from build123d import *

# Parameters (mm, degrees)
SKETCH1_W           = 116
SKETCH1_H           = 90
BOSS_EXTRUDE1_DEPTH = 5
SKETCH2_W           = 5
SKETCH2_H           = 90
BOSS_EXTRUDE2_DEPTH = 120
SKETCH3_R           = 40
CUT_EXTRUDE1_DEPTH  = 15
SKETCH4_R           = 2.5
CUT_EXTRUDE2_DEPTH  = 15
SKETCH5_W           = 5
SKETCH5_H           = 90
BOSS_EXTRUDE3_DEPTH = 120


with BuildPart() as part:
    # Sketch1 → Boss-Extrude1 (new body)
    with BuildSketch(Plane(origin=(0, 0, 0), x_dir=(1, 0, 0), z_dir=(0, 1, 0))):
        with Locations((58, 45)):
            Rectangle(SKETCH1_W, SKETCH1_H)
    extrude(amount=BOSS_EXTRUDE1_DEPTH)

    # Sketch2 → Boss-Extrude2 (add)
    with BuildSketch(Plane(origin=(0, 5, 0), x_dir=(1, 0, 0), z_dir=(0, 1, 0))):
        with Locations((113.5, 45)):
            Rectangle(SKETCH2_W, SKETCH2_H)
    extrude(amount=BOSS_EXTRUDE2_DEPTH)

    # Sketch3 → Cut-Extrude1 (cut)
    with BuildSketch(Plane.XZ):
        with Locations(Location((68, -45, 0), (0, 0, 270))):
            Circle(SKETCH3_R)
    extrude(amount=-CUT_EXTRUDE1_DEPTH, mode=Mode.SUBTRACT)

    # Sketch4 → Cut-Extrude2 (cut)
    with BuildSketch(Plane.XZ):
        with Locations(Location((32, -9, 0), (0, 0, 270))):
            Circle(SKETCH4_R)
        with Locations(Location((104, -9, 0), (0, 0, 270))):
            Circle(SKETCH4_R)
        with Locations(Location((104, -81, 0), (0, 0, 270))):
            Circle(SKETCH4_R)
        with Locations(Location((32, -81, 0), (0, 0, 270))):
            Circle(SKETCH4_R)
    extrude(amount=-CUT_EXTRUDE2_DEPTH, mode=Mode.SUBTRACT)

    # Sketch5 → Boss-Extrude3 (add)
    with BuildSketch(Plane(origin=(0, 5, 0), x_dir=(1, 0, 0), z_dir=(0, 1, 0))):
        with Locations((22.5, 45)):
            Rectangle(SKETCH5_W, SKETCH5_H)
    extrude(amount=BOSS_EXTRUDE3_DEPTH)


solid = part.part
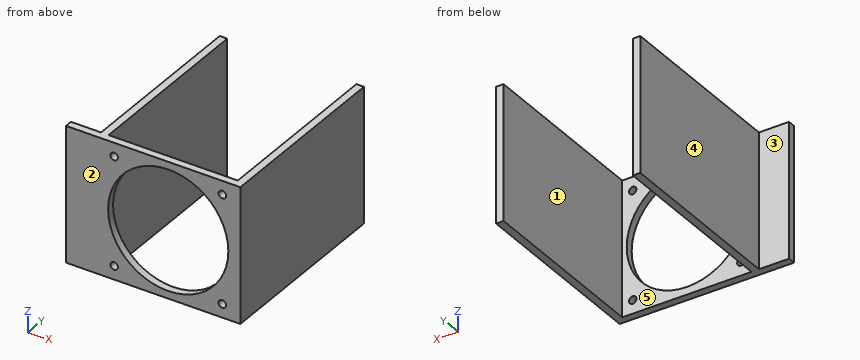
Can you work these out from the model? Positions are in its coordinate system, mm. Face numbers are marked on the shaded views. A direction names the side the tool comes from. Coordinates: 2 decimals unless noted, no trailing zeros. Loops run counter-clockwise (first coordinate to the right, second up) from the corner with the lowest first, then second, coordinate; pieces in that order, holes last. Notation, with made-up numbers: M 3.25,-35.75 L 29.25,-35.75 A20 cw 29.25,0.25 Z; hole C -7.75,82 d3. An arc over 180 degrees is marked long. Return JSON: item names as keys, results as strings. Group by question number.
Item 1: Imagine slicing it at A-A (x = 68). Please give me the cut outline in (y, z), and give its area (3 significant figures).
Item 2: Thinking about a two-plate mould opening in X: for the marked faces 3, 4 and 5, which applies, released by +X, released by -X, zero draft, split by the parting line, or undercut?
Item 3: I'm going to push flat-ended pins straight in: pin 1 Ø2 at (y, z) = (68.5, -79.5) entering from -X; pin 2 Ø8 at (x, z) = (32, -81) entering from +Y. Where does each tip first touch, or does it pass through?
Item 4: If I drill on L1, parallel to X at y = 1.3, z = -45; L2, parallel to X at y = 32.5, z = -75.5; L3, parallel to X at y = 1.55, z = -81, over which ranges is the centre line in solid material (lowest first)? Write a range as from..to.
Item 5: On a 3-axis mill with a long thin cutter (end or side, diameter ignored), from which of +Z, -Z, +X, -X, +Y, -Y can I reach the whole of each face in a straight line? I mean the marked faces 1 and 2. Say none if no direction works.
Item 6: Imagine slicing it at B-B (z = -45). Please give me the cut outline in (x, y).
Item 7: Imagine slicing it at D-D (z = -9.5). Please give me the cut outline in (x, y).
Item 8: Imagine slicing it at C-C (y = 93). Please give me the cut outline in (x, z).
Verdict:
{
 "1": {"outline": "M 0,-90 L 5,-90 L 5,-85 L 0,-85 Z; M 0,-5 L 5,-5 L 5,0 L 0,0 Z", "area": "50.0 mm^2"},
 "2": {"face 3": "zero draft", "face 4": "released by -X", "face 5": "undercut"},
 "3": {"pin 1": "stops at x = 20", "pin 2": "stops at y = 5"},
 "4": {"L1": "x = 0..28, 108..116", "L2": "x = 20..25, 111..116", "L3": "x = 0..29.5, 34.5..50.56, 85.44..101.5, 106.5..116"},
 "5": {"face 1": "+Z, -Z, +Y", "face 2": "+Z, -Z, +X, -X, -Y"},
 "6": {"outline": "M 0,0 L 28,0 L 28,5 L 25,5 L 25,125 L 20,125 L 20,5 L 0,5 Z; M 108,0 L 116,0 L 116,125 L 111,125 L 111,5 L 108,5 Z"},
 "7": {"outline": "M 0,0 L 29.55,0 L 29.55,5 L 25,5 L 25,125 L 20,125 L 20,5 L 0,5 Z; M 34.45,0 L 49.57,0 L 49.57,5 L 34.45,5 Z; M 86.43,0 L 101.55,0 L 101.55,5 L 86.43,5 Z; M 106.45,0 L 116,0 L 116,125 L 111,125 L 111,5 L 106.45,5 Z"},
 "8": {"outline": "M 20,-90 L 25,-90 L 25,0 L 20,0 Z; M 111,-90 L 116,-90 L 116,0 L 111,0 Z"}
}
